```python
from build123d import *

# Parameters (mm, degrees)
SKETCH_3_W          = 106
SKETCH_3_H          = 105
EXTRUDE_1_DEPTH     = 70
SKETCH_4_W          = 100
SKETCH_4_H          = 65
CUT_EXTRUDE_1_DEPTH = 165.805946495
FILLET_2_R          = 2.5
FILLET_3_R          = 2.5
CHAMFER_1_SIZE      = 1
SKETCH_5_W          = 2.616772355
SKETCH_5_H          = 1.7
CUT_EXTRUDE_2_DEPTH = 165.805946495
SKETCH_7_W          = 102.1
SKETCH_7_H          = 67.1
CUT_EXTRUDE_3_DEPTH = 3
FILLET_4_R          = 1
SKETCH_8_W          = 102.1
SKETCH_8_H          = 67.1
CUT_EXTRUDE_4_DEPTH = 2
FILLET_5_R          = 1
SKETCH_9_R          = 2.9
EXTRUDE_2_DEPTH     = 100
FILLET_6_R          = 1.2
SKETCH_10_R         = 1.2
CUT_EXTRUDE_5_DEPTH = 163.911018657
SKETCH_11_W         = 10
SKETCH_11_H         = 1.5
CUT_EXTRUDE_6_DEPTH = 165.805946495
SKETCH_13_W         = 0.619617199
SKETCH_13_H         = 0.675027666
SKETCH_13_H_2       = 0.576636166
SKETCH_13_W_2       = 0.693795217
SKETCH_13_W_3       = 0.795649679
EXTRUDE_3_DEPTH     = 100


with BuildPart() as part:
    # 草图3 → 凸台-拉伸1 (new body)
    with BuildSketch(Plane(origin=(0, 0, 0), x_dir=(1, 0, 0), z_dir=(0, 1, 0))):
        with Locations((53, 52.5)):
            Rectangle(SKETCH_3_W, SKETCH_3_H)
    extrude(amount=EXTRUDE_1_DEPTH)

    # 草图4 → 切除-拉伸1 (cut, through all)
    with BuildSketch(Plane.XY):
        with Locations((53, 35)):
            Rectangle(SKETCH_4_W, SKETCH_4_H)
    extrude(amount=-CUT_EXTRUDE_1_DEPTH, mode=Mode.SUBTRACT)

    # 圆角2
    fillet_2_edges = [part.edges().sort_by_distance(p)[0] for p in [
        (106, 70, -52.5),
        (0, 70, -52.5),
        (106, 0, -52.5),
        (0, 0, -52.5),
    ]]
    fillet(fillet_2_edges, radius=FILLET_2_R)

    # 圆角3
    fillet_3_edges = [part.edges().sort_by_distance(p)[0] for p in [
        (3, 2.5, -52.5),
        (3, 67.5, -52.5),
        (103, 67.5, -52.5),
        (103, 2.5, -52.5),
    ]]
    fillet(fillet_3_edges, radius=FILLET_3_R)

    # 倒角1
    chamfer_1_edges = [part.edges().sort_by_distance(p)[0] for p in [
        (106, 35, -105),
        (106, 35, 0),
        (53, 0, -105),
        (0, 35, -105),
        (53, 70, -105),
        (0.732233047, 69.267766953, -105),
        (105.267766953, 69.267766953, -105),
        (0.732233047, 0.732233047, -105),
        (105.267766953, 0.732233047, -105),
        (53, 0, 0),
        (53, 70, 0),
        (0, 35, 0),
        (0.732233047, 69.267766953, 0),
        (105.267766953, 69.267766953, 0),
        (0.732233047, 0.732233047, 0),
        (105.267766953, 0.732233047, 0),
    ]]
    chamfer(chamfer_1_edges, length=CHAMFER_1_SIZE)

    # 草图5 → 切除-拉伸2 (cut, through all)
    with BuildSketch(Plane.XY):
        with Locations((3.308386178, 10.35)):
            Rectangle(SKETCH_5_W, SKETCH_5_H)
        with Locations((102.691613823, 10.35)):
            Rectangle(SKETCH_5_W, SKETCH_5_H)
    extrude(amount=-CUT_EXTRUDE_2_DEPTH, mode=Mode.SUBTRACT)

    # 草图7 → 切除-拉伸3 (cut)
    with BuildSketch(Plane.XY):
        with Locations((53, 35)):
            Rectangle(SKETCH_7_W, SKETCH_7_H)
    extrude(amount=-CUT_EXTRUDE_3_DEPTH, mode=Mode.SUBTRACT)

    # 圆角4
    fillet_4_edges = [part.edges().sort_by_distance(p)[0] for p in [
        (1.95, 1.45, -1.5),
        (1.95, 68.55, -1.5),
        (104.05, 68.55, -1.5),
        (104.05, 1.45, -1.5),
    ]]
    fillet(fillet_4_edges, radius=FILLET_4_R)

    # 草图8 → 切除-拉伸4 (cut)
    with BuildSketch(Plane(origin=(0, 0, -105), x_dir=(-1, 0, 0), z_dir=(0, 0, -1))):
        with Locations((-53, 35)):
            Rectangle(SKETCH_8_W, SKETCH_8_H)
    extrude(amount=-CUT_EXTRUDE_4_DEPTH, mode=Mode.SUBTRACT)

    # 圆角5
    fillet_5_edges = [part.edges().sort_by_distance(p)[0] for p in [
        (104.05, 1.45, -104),
        (104.05, 68.55, -104),
        (1.95, 68.55, -104),
        (1.95, 1.45, -104),
    ]]
    fillet(fillet_5_edges, radius=FILLET_5_R)

    # 草图9 → 凸台-拉伸2 (add)
    with BuildSketch(Plane.XY.offset(-3)):
        with Locations((5.45, 4.95)):
            Circle(SKETCH_9_R)
        with Locations((100.55, 4.95)):
            Circle(SKETCH_9_R)
        with Locations((100.55, 65.05)):
            Circle(SKETCH_9_R)
        with Locations((5.45, 65.05)):
            Circle(SKETCH_9_R)
    extrude(amount=-EXTRUDE_2_DEPTH)

    # 圆角6
    fillet_6_edges = [part.edges().sort_by_distance(p)[0] for p in [
        (3, 6.501612065, -53),
        (7.001612065, 2.5, -53),
        (103, 6.501612065, -53),
        (98.998387935, 2.5, -53),
        (98.998387935, 67.5, -53),
        (103, 63.498387935, -53),
        (3, 63.498387935, -53),
        (7.001612065, 67.5, -53),
    ]]
    fillet(fillet_6_edges, radius=FILLET_6_R)

    # 草图10 → 切除-拉伸5 (cut, through all)
    with BuildSketch(Plane.XY.offset(-3)):
        with Locations((5.5, 5)):
            Circle(SKETCH_10_R)
        with Locations((100.5, 65)):
            Circle(SKETCH_10_R)
        with Locations((5.5, 65)):
            Circle(SKETCH_10_R)
        with Locations((100.5, 5)):
            Circle(SKETCH_10_R)
    extrude(amount=-CUT_EXTRUDE_5_DEPTH, mode=Mode.SUBTRACT)

    # 草图11 → 切除-拉伸6 (cut, through all)
    with BuildSketch(Plane(origin=(106, 0, 0), x_dir=(0, 0, -1), z_dir=(1, 0, 0))):
        with Locations((74, 18.75)):
            Rectangle(SKETCH_11_W, SKETCH_11_H)
        with Locations((74, 21.75)):
            Rectangle(SKETCH_11_W, SKETCH_11_H)
        with Locations((59, 18.75)):
            Rectangle(SKETCH_11_W, SKETCH_11_H)
        with Locations((59, 21.75)):
            Rectangle(SKETCH_11_W, SKETCH_11_H)
    extrude(amount=-CUT_EXTRUDE_6_DEPTH, mode=Mode.SUBTRACT)

    # 草图13 → 凸台-拉伸3 (add)
    with BuildSketch(Plane.XY.offset(-3)):
        with Locations((102.6901914, 12.069011797)):
            Rectangle(SKETCH_13_W, SKETCH_13_H)
        with Locations((102.6901914, 8.889084283)):
            Rectangle(SKETCH_13_W, SKETCH_13_H_2)
        with Locations((3.346897608, 8.889084283)):
            Rectangle(SKETCH_13_W_2, SKETCH_13_H_2)
        with Locations((3.39782484, 12.069011797)):
            Rectangle(SKETCH_13_W_3, SKETCH_13_H)
    extrude(amount=-EXTRUDE_3_DEPTH)


solid = part.part
```
Can you work these out from the model? Positions are in its coordinate system, mm. A direction names the side the tool comes from. Coordinates: 2 decimals unless noted, no trailing zeros. Loops run counter-clockwise (first coordinate to the right, second up) from the corner with the lowest first, then second, coordinate; pieces in that order, holes last. Notation, with made-up numbers: (49.25, -28) -> (73.25, -28) arc R31 cw to (73.25, 11) -> close; hole circle Ø10 at (38.25, 78). An arc over 180 degrees is marked (long way). Answer as a JSON object with one key per item and string values.
1) If I drill on line 1 (Y direction, x = 100.5, z = -35.5); line 2 (X direction, y = 65, z = -28.5); line 3 (X direction, y = 41, z = -95.5), over which ranges is the centre line in solid material (lowest first)?
Results:
{"line 1": "y = 0 to 3.8, 6.2 to 7.85, 62.15 to 63.8, 66.2 to 70", "line 2": "x = 0 to 4.3, 6.7 to 8.35, 97.65 to 99.3, 101.7 to 106", "line 3": "x = 0 to 3, 103 to 106"}
2) Imagine slicing it at C-C (z = -39). Count the separate pieces of the cut face and the enclosed holes in it, then the cut area to 3 significant figures.
Results:
{"separate pieces": "1", "enclosed holes": "5", "area": "1,000 mm^2"}
3) Thinking about a two-plate mould opening in Z: for faces 6 (the face through (52, 70, -53)), 7 (the face through (2, 19.5, -59)), 8 (the face through (1.155, 1.184, -104.618)), which applies, pulls with the +Z half, pulls with the -Z half, needs draft (parallel to the pull), parting line crosses it, or undercut?
Results:
{"face 6": "needs draft", "face 7": "undercut", "face 8": "pulls with the -Z half"}
4) Imagine slicing it at A-A (x = 89). Please give me the cut outline in (y, z), then the cut area to 4 significant figures.
Results:
{"outline": "(0, -104) -> (1, -105) -> (1.45, -105) -> (1.45, -103) -> (2.5, -103) -> (2.5, -3) -> (1.45, -3) -> (1.45, 0) -> (1, 0) -> (0, -1) -> close; (67.5, -103) -> (68.55, -103) -> (68.55, -105) -> (69, -105) -> (70, -104) -> (70, -1) -> (69, 0) -> (68.55, 0) -> (68.55, -3) -> (67.5, -3) -> close", "area": "512.5 mm^2"}
5) For P1, Ø2.5, axis at x = 105, z = -56.5, coming from the +Y side; P2, Ø2, axis at x = 5.5, y = 65, coming from the +Z side; P3, Ø0.9, axis at x = 1, z = -75, coming from the +Y side, each with a flat end and sliding along its axis, tell me the tip position at first contact or that it passes through.
Results:
{"P1": "stops at y = 69.99", "P2": "passes through", "P3": "stops at y = 69.77"}
6) For faces 1 (the face through (3, 36, -52)), 2 (the face through (98, 65, -3)), 3 (the face through (98, 65, -103)), 4 (the face through (105, 22.5, -74)), 5 (the face through (0, 35, -52)), which set-ups out of +Z, -Z, +X, -X, +Y, -Y let a thin tool reach every point of the face, with its end or its side?
Results:
{"face 1": "+Z, -Z", "face 2": "+Z", "face 3": "-Z", "face 4": "+X, -X", "face 5": "+Z, -Z, -X, +Y, -Y"}
7) Imagine slicing it at B-B (y = 26.5). Please give me the cut outline in (x, z), then the cut area to 4 significant figures.
Results:
{"outline": "(0, -104) -> (1, -105) -> (1.95, -105) -> (1.95, -103) -> (3, -103) -> (3, -3) -> (1.95, -3) -> (1.95, 0) -> (1, 0) -> (0, -1) -> close; (103, -103) -> (104.05, -103) -> (104.05, -105) -> (105, -105) -> (106, -104) -> (106, -1) -> (105, 0) -> (104.05, 0) -> (104.05, -3) -> (103, -3) -> close", "area": "617.5 mm^2"}
